from build123d import *

# Parameters (mm, degrees)
F0_W     = 16
F0_H     = 16
F0_R     = 5
F1_DEPTH = 20
F3_D     = 1.7
F3_DEPTH = 3
F3_TIP   = 0.5107315262
F5_DEPTH = 0.5


with BuildPart() as f1:
    # F0 (on Top) → F1 (new body)
    with BuildSketch(Plane.XY):
        Rectangle(F0_W, F0_H)
        Circle(F0_R, mode=Mode.SUBTRACT)
    extrude(amount=F1_DEPTH)

    # F3
    with Locations(Plane.YZ.offset(8)):
        with Locations((-5, 17), (5, 17), (5, 3), (-5, 3)):
            Hole(F3_D / 2, depth=F3_DEPTH)
            with Locations((0, 0, -(F3_DEPTH + F3_TIP / 2))):  # 118° drill point
                Cone(0, F3_D / 2, F3_TIP, mode=Mode.SUBTRACT)

    # F4 (on face) → F5 (cut)
    with BuildSketch(Plane(origin=(0, 0, 0), x_dir=(1, 0, 0), z_dir=(0, 0, -1))):
        with BuildLine():
            Line((0, -1), (6.5, -1))
            ThreePointArc((6.5, -1), (7.5, 0), (6.5, 1))
            Line((6.5, 1), (0, 1))
            Line((0, 1), (0, -1))
        make_face()
    extrude(amount=-F5_DEPTH, mode=Mode.SUBTRACT)


solid = f1.part
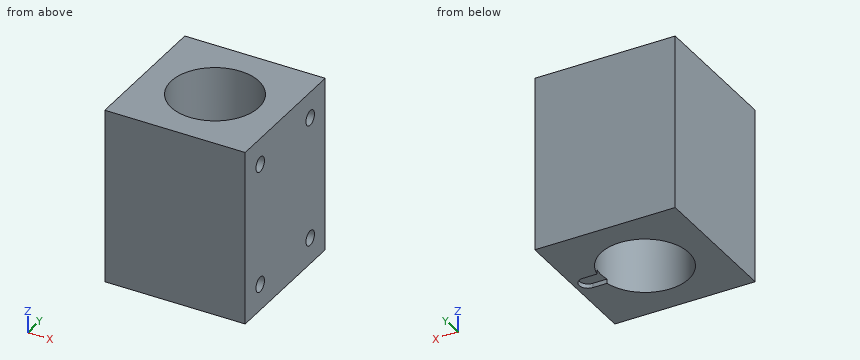
CAD build for the part. Positions are in the model's coordinates, mm. Give positions to 0.01 mm unless a question says otherwise; leave off trailing zeros. Loops run counter-clockwise (first coordinate to the right, second up) from the corner with the lowest first, then second, coordinate; pieces in that order, holes last. Notation, with made-up numbers: M -24,-8.5 L -12,-8.5 A24 ccw -12,17.5 Z; hole C 65,22 d6. An arc over 180 degrees is marked long. Answer in a Markdown table with one row per item. Add a question column.
Item 1: Drop a flat-ended pin along its axis: P1, Ø1, axis at x = 6, y = 0, coming from the -Z side. Give the stop position or say it passes through.
Item 2: Probe probe 1 along Z at (x, y) = (6, 5); probe 2 along Y at (x, z) = (5.8, 3); probe 3 along Y at (x, z) = (0, 5.5). List the from-to ranges inside material, lowest first.
Item 3: Band-saw the part on A-A on x = -3. Give the cut face in (y, z), then the cut area to 3 significant figures.
Item 4: Band-saw the part on D-D on y = 0.75. Give the cut face in (x, z), then the cut area to 3 significant figures.
Item 5: Band-saw the part on B-B on y = -2.75. Give the cut face in (x, z).
Item 6: Band-saw the part on C-C on z = 6. Give the cut face in (x, y).
Reply:
| question | item | result |
|---|---|---|
| 1 | P1 | stops at z = 0.5 |
| 2 | probe 1 | z = 0 to 2.15, 3.85 to 16.15, 17.85 to 20 |
| 2 | probe 2 | y = -8 to -5.85, -4.15 to 4.15, 5.85 to 8 |
| 2 | probe 3 | y = -8 to -5, 5 to 8 |
| 3 | outline | M -8,0 L -4,0 L -4,20 L -8,20 Z; M 4,0 L 8,0 L 8,20 L 4,20 Z |
| 3 | area | 160 mm^2 |
| 4 | outline | M -8,0 L -4.94,0 L -4.94,20 L -8,20 Z; M 4.94,0.5 L 7.16,0.5 L 7.16,0 L 8,0 L 8,20 L 4.94,20 Z |
| 4 | area | 121 mm^2 |
| 5 | outline | M -8,0 L -4.18,0 L -4.18,20 L -8,20 Z; M 4.18,0 L 8,0 L 8,20 L 4.18,20 Z |
| 6 | outline | M -8,-8 L 8,-8 L 8,8 L -8,8 Z; hole C 0,0 d10 |
